Geometry check sheet. Reference: the model listing, model coordinates, mm. Face numbers are marked on the shaded views. A direction names the side the tool comes from. Round coordinates to 2 decimals unless told otherwise and drop trailing zeros. Order: outer loops, then holes, each group sorted by start corner. A loop starts at its lowest first (then second) coordinate and runs counter-clockwise, first axis right, second up. Notation, with made-up numbers: (67.5, 55) - (117.5, 55) arc R14 cw to (117.5, 64) - close; hole circle Ø9 at (89, 57). An arc over 180 degrees is marked (long way). One line per question, with ' | ' between items. Start each with the question number.
Q1. Gauge pin test, flat ends, axial feed: P1, Ø1.5, axis at y = -33, z = 29.5, coming from the -X side; P2, Ø4, axis at y = -31.5, z = 32, coming from the +X side; P3, Ø2.5, axis at x = 64, z = 23.5, coming from the -Y side; P4, Ø2.5, axis at x = 134.49, z = 45.51, coming from the +Y side. Record the tip position at first contact, or that the pin passes through.
Q2. Tool access check on the marked faces 1, 2 and 3. Record the directions out of +Z, -Z, +X, -X, +Y, -Y that give a thin tool (end or side, any length) a straight path to the whole face; none if there is none.
Q3. Sectioned sample at A-A, the plane y = -32. Give the number of separate pieces and of enclosed holes in the cut face, then the cut area to 3 significant figures.
Q4. Sectioned sample at C-C, the plane y = -14.5. Enter the section's corners in (x, z), then the cut area to 3 significant figures.
Q5. Material ranges on line 1 along X through (y, z) = (-2, 9.5); line 2 along Z through (x, y) = (35, -32); line 3 along Y through (x, z) = (13, 35.5), recorded low to high.
Q6. Sectioned sample at B-B, the plane x = 121. Enter the section's corners in (y, z).
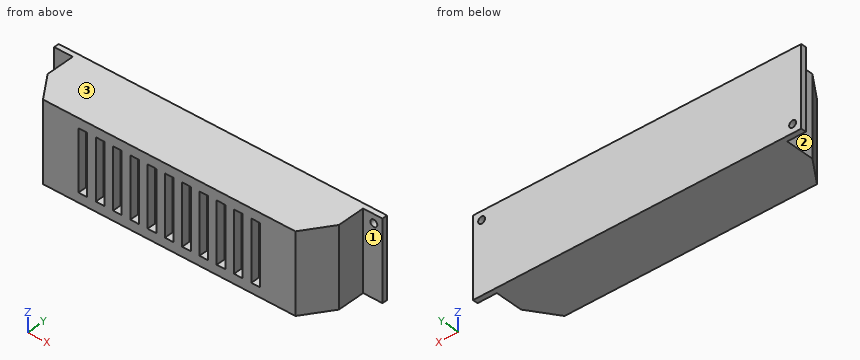
Solid Edge part; units mm, degrees
sketch "Sketch1" plane through (0, 0, 0) normal (0, -1, 0) x (1, 0, 0)
  line L0 (-50.5116, 4.5081) -> (139.4884, 4.5081)
  line L1 (139.4884, 4.5081) -> (139.4884, 50.5081)
  line L2 (139.4884, 50.5081) -> (-50.5116, 50.5081)
  line L3 (-50.5116, 50.5081) -> (-50.5116, 4.5081)
  circle A0 centre (-45.5116, 9.5081) radius 2
  circle A1 centre (134.4884, 45.5081) radius 2
extrude "Protrusion1" add sketch "Sketch1" along normal blind 35
sketch "Sketch2" plane through (44.4884, -17.5, 4.5081) normal (0, 0, -1) x (1, 0, 0)
  line L0 (-95, -17.5) -> (-95, -14.5)
  line L1 (-95, -14.5) -> (-84.26, -14.5)
  line L2 (-84.26, -14.5) -> (-84.26, 2.1617)
  line L3 (-84.26, 2.1617) -> (-73.52, 17.5)
  line L4 (72.5934, 17.5) -> (-73.52, 17.5)
  line L5 (83.7967, 1.5) -> (72.5934, 17.5)
  line L6 (83.7967, -14.5) -> (83.7967, 1.5)
  line L7 (95, -14.5) -> (83.7967, -14.5)
  line L8 (95, -17.5) -> (95, -14.5)
  line L9 (100.6753, -17.5) -> (95, -17.5)
  line L10 (100.6753, 23.6883) -> (100.6753, -17.5)
  line L11 (-100.9714, 23.6883) -> (100.6753, 23.6883)
  line L12 (-100.9714, -17.5) -> (-100.9714, 23.6883)
  line L13 (-95, -17.5) -> (-100.9714, -17.5)
extrude "ExtrudedCutout_1" cut sketch "Sketch2" against normal blind 46
sketch "Sketch3" plane through (44.025, -35, 27.5081) normal (0, -1, 0) x (1, 0, 0)
  line L0 (-2.5, -17.5) -> (2.5, -17.5)
  line L1 (2.5, -17.5) -> (2.5, 17.5)
  line L2 (2.5, 17.5) -> (-2.5, 17.5)
  line L3 (-2.5, 17.5) -> (-2.5, -17.5)
  line L4 (7.5, -17.5) -> (12.5, -17.5)
  line L5 (12.5, -17.5) -> (12.5, 17.5)
  line L6 (12.5, 17.5) -> (7.5, 17.5)
  line L7 (7.5, 17.5) -> (7.5, -17.5)
  line L8 (17.5, -17.5) -> (22.5, -17.5)
  line L9 (22.5, -17.5) -> (22.5, 17.5)
  line L10 (22.5, 17.5) -> (17.5, 17.5)
  line L11 (17.5, 17.5) -> (17.5, -17.5)
  line L12 (27.5, -17.5) -> (32.5, -17.5)
  line L13 (32.5, -17.5) -> (32.5, 17.5)
  line L14 (32.5, 17.5) -> (27.5, 17.5)
  line L15 (27.5, 17.5) -> (27.5, -17.5)
  line L16 (37.5, -17.5) -> (42.5, -17.5)
  line L17 (42.5, -17.5) -> (42.5, 17.5)
  line L18 (42.5, 17.5) -> (37.5, 17.5)
  line L19 (37.5, 17.5) -> (37.5, -17.5)
  line L20 (-12.5, -17.5) -> (-7.5, -17.5)
  line L21 (-7.5, -17.5) -> (-7.5, 17.5)
  line L22 (-7.5, 17.5) -> (-12.5, 17.5)
  line L23 (-12.5, 17.5) -> (-12.5, -17.5)
  line L24 (-22.5, -17.5) -> (-17.5, -17.5)
  line L25 (-17.5, -17.5) -> (-17.5, 17.5)
  line L26 (-17.5, 17.5) -> (-22.5, 17.5)
  line L27 (-22.5, 17.5) -> (-22.5, -17.5)
  line L28 (-32.5, -17.5) -> (-27.5, -17.5)
  line L29 (-27.5, -17.5) -> (-27.5, 17.5)
  line L30 (-27.5, 17.5) -> (-32.5, 17.5)
  line L31 (-32.5, 17.5) -> (-32.5, -17.5)
  line L32 (-42.5, -17.5) -> (-37.5, -17.5)
  line L33 (-37.5, -17.5) -> (-37.5, 17.5)
  line L34 (-37.5, 17.5) -> (-42.5, 17.5)
  line L35 (-42.5, 17.5) -> (-42.5, -17.5)
  line L36 (-52.5, -17.5) -> (-47.5, -17.5)
  line L37 (-47.5, -17.5) -> (-47.5, 17.5)
  line L38 (-47.5, 17.5) -> (-52.5, 17.5)
  line L39 (-52.5, 17.5) -> (-52.5, -17.5)
  line L40 (47.5, -17.5) -> (52.5, -17.5)
  line L41 (52.5, -17.5) -> (52.5, 17.5)
  line L42 (52.5, 17.5) -> (47.5, 17.5)
  line L43 (47.5, 17.5) -> (47.5, -17.5)
extrude "ExtrudedCutout_2" cut sketch "Sketch3" against normal blind 5
Determined:
1) P1: stops at x = -30.96 | P2: stops at x = 120.93 | P3: stops at y = -30 | P4: passes through
2) face 1: +Z, -Z, +X, -Y | face 2: +Z, -Z, -X, -Y | face 3: +Z, +X, -X, +Y, -Y
3) separate pieces: 1 | enclosed holes: 11 | area: 4,990 mm2
4) outline: (-39.77, 4.51) - (128.29, 4.51) - (128.29, 50.51) - (-39.77, 50.51) - close | area: 7,730 mm2
5) line 1: x = -50.51 to -47.51, -43.51 to 139.49 | line 2: z = 4.51 to 10.01, 45.01 to 50.51 | line 3: y = -30 to 0
6) outline: (-29.4, 4.51) - (0, 4.51) - (0, 50.51) - (-29.4, 50.51) - close
